The listing builds one solid part. Answer for the finished solid, in the listing's coordinates (mm). A direction names the side the tool comes from. Coordinates: 2 decimals unless noted, no trailing zeros. Order: outer loops, then holes, each group sorted by start corner. A loop starts at its lowest first (then second) coordinate and runs counter-clockwise, first axis right, second up. Notation, with made-up numbers: (-6, 6) -> (42, 6) arc R12 cw to (42, 28) -> close; hole circle Ø1 at (-8.5, -29.75). An arc over 180 degrees is marked (long way). Answer in a Markdown table with one row per item.
```python
from build123d import *

# Parameters (mm, degrees)
SKETCH_1_W          = 4.2
SKETCH_1_H          = 49
EXTRUDE_1_DEPTH     = 5
SKETCH_5_R          = 1.65
CUT_EXTRUDE_2_DEPTH = 5
SKETCH_6_W          = 4.2
SKETCH_6_H          = 3
EXTRUDE_2_DEPTH     = 59
SKETCH_11_R         = 1.65
EXTRUDE_3_DEPTH     = 3
SKETCH_12_W         = 6.956074108
SKETCH_12_H         = 25
CUT_EXTRUDE_3_DEPTH = 10


with BuildPart() as part:
    # 草图1 → 凸台-拉伸1 (new body)
    with BuildSketch(Plane.XY):
        with Locations((2.1, -24.5)):
            Rectangle(SKETCH_1_W, SKETCH_1_H)
    extrude(amount=EXTRUDE_1_DEPTH)

    # 草图5 → 切除-拉伸2 (cut)
    with BuildSketch(Plane.XY.offset(5)):
        with Locations((2.1, -9)):
            Circle(SKETCH_5_R)
        with Locations(Location((2.1, -40, 0), (0, 0, 180))):
            Circle(SKETCH_5_R)
    extrude(amount=-CUT_EXTRUDE_2_DEPTH, mode=Mode.SUBTRACT)

    # 草图6 → 凸台-拉伸2 (add)
    with BuildSketch(Plane.XY.offset(5)):
        with Locations((2.1, -50.5)):
            Rectangle(SKETCH_6_W, SKETCH_6_H)
        with Locations((2.1, 1.5)):
            Rectangle(SKETCH_6_W, SKETCH_6_H)
    extrude(amount=-EXTRUDE_2_DEPTH)

    # 草图11 → 凸台-拉伸3 (add)
    # profile 1 of 2: a face of its own
    with BuildSketch(Plane(origin=(0, 0, -54), x_dir=(-1, 0, 0), z_dir=(0, 0, -1))):
        Polygon((-2.1, 3), (-5.1, 3), (-5.1, 10), (0, 10), (0, 3), align=None)
        with Locations((-2.1, 7)):
            Circle(SKETCH_11_R, mode=Mode.SUBTRACT)
    # profile 2 of 2: a face of its own
    with BuildSketch(Plane(origin=(0, 0, -54), x_dir=(-1, 0, 0), z_dir=(0, 0, -1))):
        Polygon((0, -59), (-5.1, -59), (-5.1, -52), (-2.1, -52), (0, -52), align=None)
        with Locations(Location((-2.1, -56, 0), (0, 0, 180))):
            Circle(SKETCH_11_R, mode=Mode.SUBTRACT)
    extrude(amount=-EXTRUDE_3_DEPTH)

    # 草图12 → 切除-拉伸3 (cut)
    with BuildSketch(Plane.XY.offset(5)):
        with Locations((5.578037054, -24.5)):
            Rectangle(SKETCH_12_W, SKETCH_12_H)
    extrude(amount=-CUT_EXTRUDE_3_DEPTH, mode=Mode.SUBTRACT)


solid = part.part
```
(1) A cutting plane is placed at C-C, the plane y = -53.5. Determine the outline of the cut face in (x, z).
Check values:
| item | result |
|---|---|
| outline | (0, -54) -> (5.1, -54) -> (5.1, -51) -> (0, -51) -> close |
(2) For a pull along Y with two mould halves and no side action, classify faces 4 (the flat face through (2, -49, -27)), 5 (the flat face through (3, -59, -53)), 6 (the flat face through (5.1, 6, -53)) as released by +Y, released by -Y, zero draft, split by the parting line, or undercut.
Check values:
| item | result |
|---|---|
| face 4 | undercut |
| face 5 | released by -Y |
| face 6 | zero draft |
(3) A cutting plane is placed at B-B, the plane z = -1. Determine the outline of the cut face in (x, y), then the cut area to 3 significant figures.
Check values:
| item | result |
|---|---|
| outline | (0, -52) -> (4.2, -52) -> (4.2, -49) -> (0, -49) -> close; (0, 0) -> (4.2, 0) -> (4.2, 3) -> (0, 3) -> close |
| area | 25.2 mm² |
(4) A cutting plane is placed at D-D, the plane y = -16. Determine the outline of the cut face in (x, z).
Check values:
| item | result |
|---|---|
| outline | (0, 0) -> (2.1, 0) -> (2.1, 5) -> (0, 5) -> close |
(5) Which of the six approach directions +Z, -Z, +X, -X, +Y, -Y give full straight-line access (tool end or side, diameter ignored) to faces 1 (the flat face through (4, -55, -51)), 2 (the flat face through (2, 0, -27)), 3 (the flat face through (2.1, -25, 3))?
Check values:
| item | result |
|---|---|
| face 1 | +Z, +X, -X, -Y |
| face 2 | -Z, +X, -X |
| face 3 | +Z, -Z, +X |
(6) Flat-ended cylindrical pins translate along their axes: pin 1 (1.3 mm diameter, centred on x = 3, z = -11, fed in from -Y); pin 2 (1.7 mm diameter, centred on x = 2.5, z = 1.5, fed in from +Y); pin 3 (1.5 mm diameter, centred on x = 3, y = -15, fed in from +Z); pin 4 (5 mm diameter, centred on y = -52, z = -29, fed in from +X). Find the tip coordinate at first contact, or state that the pin passes through.
Check values:
| item | result |
|---|---|
| pin 1 | y = -52 |
| pin 2 | y = 3 |
| pin 3 | through |
| pin 4 | x = 4.2 |
(7) A cutting plane is placed at A-A, the plane y = -9. Determine the outline of the cut face in (x, z), then the cut area to 3 significant figures.
Check values:
| item | result |
|---|---|
| outline | (0, 0) -> (0.45, 0) -> (0.45, 5) -> (0, 5) -> close; (3.75, 0) -> (4.2, 0) -> (4.2, 5) -> (3.75, 5) -> close |
| area | 4.50 mm² |
(8) Find the intervals of material crossed by line 1 along Y through (x, z) = (2.6, -49); line 2 along X through (y, z) = (-56, -52.45); line 3 along Z through (x, y) = (2.35, 5), in increasing order. Write a range as from..to.
Check values:
| item | result |
|---|---|
| line 1 | -52..-49, 0..3 |
| line 2 | 0..0.45, 3.75..5.1 |
| line 3 | -54..-51 |
